Read the model definition and answer for the solid it produces. Units are mm, in the model's axes. Give positions to 0.01 mm unless a question says otherwise; leave off trailing zeros. Write each loop counter-clockwise with the first axis right and the second up, starting at its lowest first coordinate (ties: lowest second). Pieces come first, ordered by that corner, then holes. Notation, with made-up numbers: (0.25, 42.25) -> (53.25, 42.25) arc R19 cw to (53.25, 47.25) -> close; hole circle Ø10 at (39.5, 7.25). An arc over 180 degrees is marked (long way). Use a Markdown table: item, result.
from build123d import *

# Parameters (mm, degrees)
ESQUISSE1_W             = 150
ESQUISSE1_H             = 210
BOSS_EXTRU_1_DEPTH      = 5
D_GAGEMENT_M81_D        = 9
ESQUISSE5_W             = 40
ESQUISSE5_H             = 30
ENL_V_MAT_EXTRU_1_DEPTH = 5
ENL_V_MAT_EXTRU_2_DEPTH = 5
ESQUISSE7_R             = 48.156846138
ENL_V_MAT_EXTRU_3_DEPTH = 5


with BuildPart() as part:
    # Esquisse1 → Boss.-Extru.1 (new body)
    with BuildSketch(Plane.XY):
        with Locations((75, -105)):
            Rectangle(ESQUISSE1_W, ESQUISSE1_H)
    extrude(amount=BOSS_EXTRU_1_DEPTH)

    # Dégagement M81 (through all)
    with Locations(Plane.XY.offset(5)):
        with Locations((85, -23.12089623), (85, -143.12089623), (15, -143.12089623), (15, -39.62089623)):
            Hole(D_GAGEMENT_M81_D / 2)

    # Esquisse5 → Enlèv. mat.-Extru.1 (cut)
    with BuildSketch(Plane.XY.offset(5)):
        with Locations((78, -172.12089623)):
            Rectangle(ESQUISSE5_W, ESQUISSE5_H)
    extrude(amount=-ENL_V_MAT_EXTRU_1_DEPTH, mode=Mode.SUBTRACT)

    # Esquisse6 → Enlèv. mat.-Extru.2 (cut)
    with BuildSketch(Plane.XY.offset(5)):
        Polygon((0, -210), (0, -150), (70, -210), align=None)
    extrude(amount=-ENL_V_MAT_EXTRU_2_DEPTH, mode=Mode.SUBTRACT)

    # Esquisse7 → Enlèv. mat.-Extru.3 (cut)
    with BuildSketch(Plane.XY.offset(5)):
        with Locations((70.667772287, -83.194453846)):
            Circle(ESQUISSE7_R)
    extrude(amount=-ENL_V_MAT_EXTRU_3_DEPTH, mode=Mode.SUBTRACT)


solid = part.part
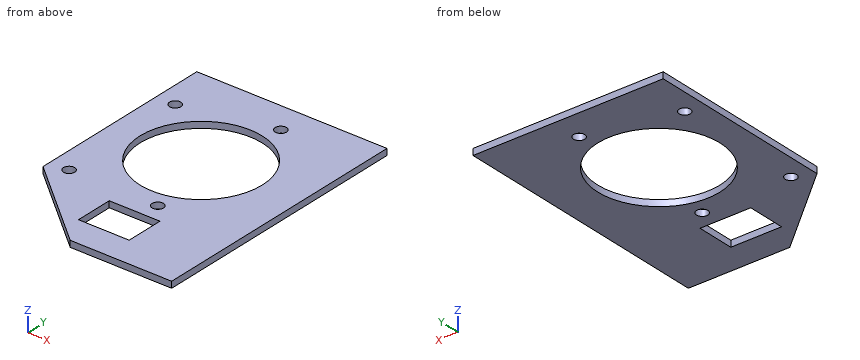
Item 1: A cutting plane is placed at A-A (x = 85). Give the vertices of the cut face in (y, z).
Return value:
| item | result |
|---|---|
| outline | (-210, 0) -> (-187.12, 0) -> (-187.12, 5) -> (-210, 5) -> close; (-157.12, 0) -> (-147.62, 0) -> (-147.62, 5) -> (-157.12, 5) -> close; (-138.62, 0) -> (-129.17, 0) -> (-129.17, 5) -> (-138.62, 5) -> close; (-37.22, 0) -> (-27.62, 0) -> (-27.62, 5) -> (-37.22, 5) -> close; (-18.62, 0) -> (0, 0) -> (0, 5) -> (-18.62, 5) -> close |
Item 2: A cutting plane is placed at D-D (z = 4.1). Give the vertices of the cut face in (x, y), then the cut area to 3 significant figures.
Return value:
| item | result |
|---|---|
| outline | (0, -150) -> (70, -210) -> (150, -210) -> (150, 0) -> (0, 0) -> close; hole circle Ø9 at (15, -143.12); hole circle Ø9 at (15, -39.62); hole circle Ø96.31 at (70.67, -83.19); hole (58, -187.12) -> (98, -187.12) -> (98, -157.12) -> (58, -157.12) -> close; hole circle Ø9 at (85, -143.12); hole circle Ø9 at (85, -23.12) |
| area | 20,700 mm^2 |
Item 3: A cutting plane is placed at B-B (y = -121.5). Give the vertices of the cut face in (x, z).
Return value:
| item | result |
|---|---|
| outline | (0, 0) -> (41.48, 0) -> (41.48, 5) -> (0, 5) -> close; (99.85, 0) -> (150, 0) -> (150, 5) -> (99.85, 5) -> close |
Item 4: A cutting plane is placed at C-C (x = 25.5). Give the vertices of the cut face in (y, z), then the cut area to 3 significant figures.
Return value:
| item | result |
|---|---|
| outline | (-171.86, 0) -> (-99.9, 0) -> (-99.9, 5) -> (-171.86, 5) -> close; (-66.49, 0) -> (0, 0) -> (0, 5) -> (-66.49, 5) -> close |
| area | 692 mm^2 |
Item 5: This flat-tipped pin is pushed along its axis until it touches: P1, Ø2, axis at y = -108, z = 1.5, coming from the -X side. Where does it stop, or does it pass through?
Return value:
| item | result |
|---|---|
| P1 | x = 0 |
Item 6: Straight lines are drawn through the part: line 1 along Y through (x, z) = (70, 4.8); line 2 along X through (y, z) = (-142.5, 4.6); line 3 along Y through (x, z) = (87, 3.45). For each, find the intervals that lie inside material, in ascending order. Write a range as [from, to].
Return value:
| item | result |
|---|---|
| line 1 | [-210, -187.12], [-157.12, -131.35], [-35.04, 0] |
| line 2 | [0, 10.54], [19.46, 80.54], [89.46, 150] |
| line 3 | [-210, -187.12], [-157.12, -147.15], [-139.09, -128.5], [-37.89, -27.15], [-19.09, 0] |
